from build123d import *

# Parameters (mm, degrees)
IZIM1_W                     = 27
IZIM1_H                     = 96
IZIM1_R                     = 1.5
IZIM1_R_2                   = 2
Y_KSEKLIK_EKSTR_ZYON1_DEPTH = 1
IZGIDEN_START               = 367.447539798
IZGIDEN_B_KME1_OUTLINE_W    = 96
IZGIDEN_B_KME1_OUTLINE_H    = 1
IZGIDEN_B_KME1_DEPTH        = 32.552460202
IZGIDEN_START_2             = 365.658779798
IZGIDEN_B_KME1_2_OUTLINE_R  = 2
IZGIDEN_B_KME1_2_DEPTH      = 2
IZGIDEN_START_3             = -15.757423971
IZGIDEN_B_KME1_3_DEPTH      = 96


with BuildPart() as part:
    # Çizim1 → Yükseklik-Ekstrüzyon1 (new body)
    # profile 1 of 2: a face of its own
    with BuildSketch(Plane.XY):
        with Locations((353.158779798, 32.242576029)):
            Rectangle(IZIM1_W, IZIM1_H)
        with Locations((344.658779798, -4.257423971)):
            Circle(IZIM1_R, mode=Mode.SUBTRACT)
        with Locations((344.658779798, 68.742576029)):
            Circle(IZIM1_R, mode=Mode.SUBTRACT)
    # profile 2 of 2: a face of its own
    with BuildSketch(Plane.XY):
        with BuildLine():
            Line((376.658779798, 80.242576029), (366.658779798, 80.242576029))
            Line((366.658779798, 80.242576029), (366.658779798, -15.757423971))
            Line((366.658779798, -15.757423971), (376.658779798, -15.757423971))
            ThreePointArc((376.658779798, -15.757423971), (399.170626089, 32.242576029), (376.658779798, 80.242576029))
        make_face()
        with Locations((382.658779798, 16.742576029)):
            Circle(IZIM1_R_2, mode=Mode.SUBTRACT)
        with Locations((382.658779798, 47.742576029)):
            Circle(IZIM1_R_2, mode=Mode.SUBTRACT)
    extrude(amount=Y_KSEKLIK_EKSTR_ZYON1_DEPTH)

    # Çizgiden Bükme1: read off the stored shape, not the designer's step
    # Çizgiden Bükme1 outline → Çizgiden Bükme1 (cut)
    with BuildSketch(Plane.YZ.offset(IZGIDEN_START)):
        with Locations((32.242576029, 0.5)):
            Rectangle(IZGIDEN_B_KME1_OUTLINE_W, IZGIDEN_B_KME1_OUTLINE_H)
    extrude(amount=IZGIDEN_B_KME1_DEPTH, mode=Mode.SUBTRACT)

    # izgiden B_kme1 2 outline → izgiden B_kme1 2 (add)
    with BuildSketch(Plane.YZ.offset(IZGIDEN_START_2)):
        with BuildLine():
            Line((80.242576029, 1), (80.242576029, 10.64380551))
            ThreePointArc((80.242576029, 10.64380551), (32.242576029, 33.155651801), (-15.757423971, 10.64380551))
            Line((-15.757423971, 10.64380551), (-15.757423971, 1))
            Line((-15.757423971, 1), (80.242576029, 1))
        make_face()
        with Locations((16.742576029, 16.64380551)):
            Circle(IZGIDEN_B_KME1_2_OUTLINE_R, mode=Mode.SUBTRACT)
        with Locations((47.742576029, 16.64380551)):
            Circle(IZGIDEN_B_KME1_2_OUTLINE_R, mode=Mode.SUBTRACT)
    extrude(amount=IZGIDEN_B_KME1_2_DEPTH)

    # izgiden B_kme1 3 outline → izgiden B_kme1 3 (cut)
    with BuildSketch(Plane(origin=(0, 0, 0), x_dir=(1, 0, 0), z_dir=(0, 1, 0)).offset(IZGIDEN_START_3)):
        with BuildLine():
            Line((366.658779798, -35), (366.658779798, -2))
            ThreePointArc((366.658779798, -2), (366.365886579, -1.292893219), (365.658779798, -1))
            Line((365.658779798, -1), (365.658779798, -35))
            Line((365.658779798, -35), (366.658779798, -35))
        make_face()
        with BuildLine():
            Line((367.658779798, -2), (367.658779819, -35))
            Line((367.658779819, -35), (369, -35))
            Line((369, -35), (369, -1))
            Line((369, -1), (367.447539798, -1))
            Line((367.447539798, -1), (367.447539798, 1))
            Line((367.447539798, 1), (364, 1))
            Line((364, 1), (364, 1e-09))
            Line((364, 1e-09), (365.658779798, 0))
            ThreePointArc((365.658779798, 0), (367.07299336, -0.585786438), (367.658779798, -2))
        make_face()
    extrude(amount=IZGIDEN_B_KME1_3_DEPTH, mode=Mode.SUBTRACT)


solid = part.part
Verification items for the finished model (mm, model axes). A direction names the side the tool comes from. Coordinates: 2 decimals unless noted, no trailing zeros. Write each loop counter-clockwise with the first axis right and the second up, starting at its lowest first coordinate (ties: lowest second). Pieces come first, ordered by that corner, then holes. Notation, with made-up numbers: M 72.25,30 L 81.25,30 A26 cw 81.25,65 Z; hole C 3,17 d11. An arc over 180 degrees is marked long. Use a Markdown table: item, result.
Q1. Sectioned sample at D-D, the plane y = 4.5. Record the boundary of the cut face in (x, z), plus the area to 3 significant figures.
Reply:
| item | result |
|---|---|
| outline | M 339.66,0 L 365.66,0 A2 ccw 367.66,2 L 367.66,26.65 L 366.66,26.65 L 366.66,2 A1 cw 365.66,1 L 339.66,1 Z |
| area | 53.0 mm² |
Q2. Sectioned sample at A-A, the plane x = 345. Record the boundary of the cut face in (y, z).
Reply:
| item | result |
|---|---|
| outline | M -15.76,0 L -5.72,0 L -5.72,1 L -15.76,1 Z; M -2.8,0 L 67.28,0 L 67.28,1 L -2.8,1 Z; M 70.2,0 L 80.24,0 L 80.24,1 L 70.2,1 Z |
Q3. Go/stop test with flat-tipped pins: P1, Ø3.5, axis at x = 344.66, y = 68.74, coming from the +Z side; P2, Ø6, axis at y = 44, z = 11, coming from the -X side. Record where each tip stops, or that it passes through.
Reply:
| item | result |
|---|---|
| P1 | stops at z = 1 |
| P2 | stops at x = 366.66 |
Q4. Draft check along Z on faces 1 (the face through (357.7, -15.757, 0.6)), 2 (the face through (367.15, 49.65, 17.24)), 3 (the face through (367.057, 31.571, 0.57)). Enter one of: +Z half, -Z half, draft (parallel to the pull), parting line (faces both ways), or undercut.
Reply:
| item | result |
|---|---|
| face 1 | draft |
| face 2 | undercut |
| face 3 | -Z half |
Q5. Set-up check for faces 4 (the face through (343.553, -3.244, 0.493)), 5 (the face through (352, 33, 1)): record each of +Z, -Z, +X, -X, +Y, -Y from which the full face is reachable in a straight line by a thin tool's end or side.
Reply:
| item | result |
|---|---|
| face 4 | +Z, -Z |
| face 5 | +Z, -X, +Y, -Y |
Q6. Sectioned sample at C-C, the plane z = 7. Record the boundary of the cut face in (x, y), plus the area to 3 significant figures.
Reply:
| item | result |
|---|---|
| outline | M 366.66,-15.76 L 367.66,-15.76 L 367.66,80.24 L 366.66,80.24 Z |
| area | 96.0 mm² |
Q7. Thickness scan on line 1 (X direction, y = 42.5, z = 29); line 2 (Z direction, x = 358, y = 64.5). Record the ranges inside material, lowest first.
Reply:
| item | result |
|---|---|
| line 1 | x = 366.66 to 367.66 |
| line 2 | z = 0 to 1 |
Q8. Sectioned sample at B-B, the plane y = 47. Record the boundary of the cut face in (x, z).
Reply:
| item | result |
|---|---|
| outline | M 339.66,0 L 365.66,0 A2 ccw 367.66,2 L 367.66,14.79 L 366.66,14.79 L 366.66,2 A1 cw 365.66,1 L 339.66,1 Z; M 366.66,18.5 L 367.66,18.5 L 367.66,31.39 L 366.66,31.39 Z |
